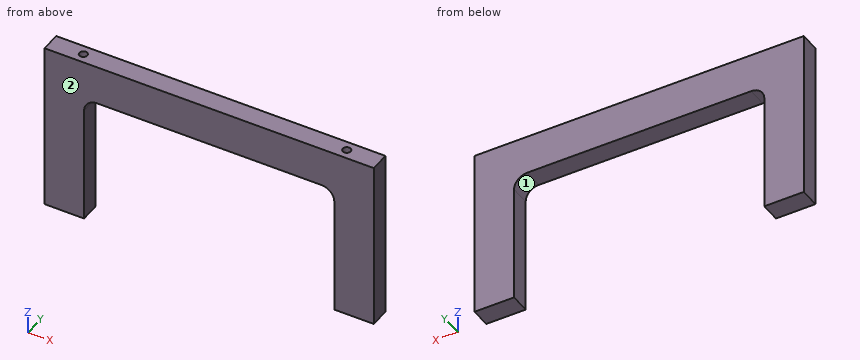
from build123d import *

# Parameters (mm, degrees)
F0_W     = 250
F0_H     = 15
F1_DEPTH = 130
F2_D     = 6
F2_DEPTH = 7
F2_TIP   = 1.8025818571
F4_DEPTH = 12.5


with BuildPart() as f1:
    # F0 (on Top) → F1 (new body)
    with BuildSketch(Plane.XY):
        Rectangle(F0_W, F0_H)
    extrude(amount=-F1_DEPTH)

    # F2
    with Locations(Plane.XY):
        with Locations((-100, 0), (100, 0)):
            Hole(F2_D / 2, depth=F2_DEPTH)
            with Locations((0, 0, -(F2_DEPTH + F2_TIP / 2))):  # 118° drill point
                Cone(0, F2_D / 2, F2_TIP, mode=Mode.SUBTRACT)

    # F3 (on Front) → F4 (cut, symmetric)
    with BuildSketch(Plane.XZ):
        with BuildLine():
            Line((-95, -177.2061562841), (95, -177.2061562841))
            Line((95, -177.2061562841), (95, -40))
            ThreePointArc((95, -40), (92.0710678119, -32.9289321881), (85, -30))
            Line((85, -30), (-85, -30))
            ThreePointArc((-85, -30), (-92.0710678119, -32.9289321881), (-95, -40))
            Line((-95, -40), (-95, -177.2061562841))
        make_face()
    extrude(amount=F4_DEPTH, both=True, mode=Mode.SUBTRACT)


solid = f1.part
Model file for the job. Use its own axes, mm. Face numbers are marked on the shaded views. A direction names the side the tool comes from. Give positions to 0.01 mm unless a question says otherwise; leave off trailing zeros. Write each loop counter-clockwise with the first axis right and the second up, starting at its lowest first coordinate (ties: lowest second). Pieces come first, ordered by that corner, then holes. Notation, with made-up numbers: M 86.25,2.25 L 140.25,2.25 A30 cw 140.25,29.25 Z; hole C 42.25,54 d3. An arc over 180 degrees is marked long. One line per item, written item: value. Start each with the question number.
Q1. Saw through at B-B, the plane x = -80. Write the cut outline in (y, z), plus the area to 3 significant figures.
Q2. 3-axis set-ups, long thin cutter, end or side, ignore diameter. For the marked faces 1 and 2: which of +Z, -Z, +X, -X, +Y, -Y reach the whole face in a straight line?
Q3. Drop flat-ended pins along their axis: pin 1 Ø6 at (x, y) = (77.5, -1.5) entering from -Z; pin 2 Ø8 at (x, y) = (-2.5, 5.5) entering from +Z; pin 3 Ø5.5 at (x, y) = (-100, 0) entering from +Z. Give the stop position or say it passes through.
Q4. Saw through at A-A, the plane z = -55.5. Write the cut outline in (x, y), plus the area to 3 significant figures.
Q5. Probe probe 1 along X at (y, z) = (0, -1.25); probe 2 along Y at (x, z) = (-100, -5); probe 3 along X at (y, z) = (-1, -112). List the from-to ranges inside material, lowest first. Write a range as [from, to].
Output values:
1. outline: M -7.5,-30 L 7.5,-30 L 7.5,0 L -7.5,0 Z
1. area: 450 mm²
2. face 1: -Z, +Y, -Y
2. face 2: +Z, -Z, +X, -X, -Y
3. pin 1: stops at z = -30
3. pin 2: stops at z = 0
3. pin 3: stops at z = -7.15
4. outline: M -125,-7.5 L -95,-7.5 L -95,7.5 L -125,7.5 Z; M 95,-7.5 L 125,-7.5 L 125,7.5 L 95,7.5 Z
4. area: 900 mm²
5. probe 1: x = [-125, -103], [-97, 97], [103, 125]
5. probe 2: y = [-7.5, -3], [3, 7.5]
5. probe 3: x = [-125, -95], [95, 125]
